Geometry check sheet. Reference: the model listing, model coordinates, mm. Face numbers are marked on the shaded views. A direction names the side the tool comes from. Coordinates: 2 decimals unless noted, no trailing zeros. Loops run counter-clockwise (first coordinate to the right, second up) from the corner with the lowest first, then second, coordinate; pieces in that order, holes last. Notation, with made-up numbers: (10.5, 20.25) - (24.5, 20.25) arc R26 ccw to (24.5, 38.25) - close; hole circle Ø9 at (6, -25.5). An arc over 180 degrees is marked (long way). One line per item, written item: value.
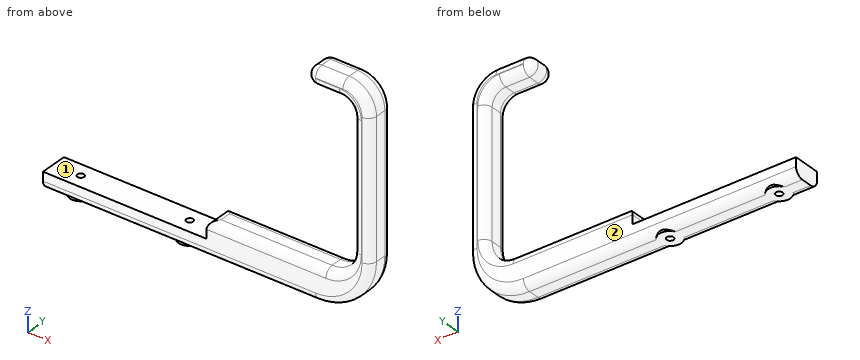
from build123d import *

# Parameters (mm, degrees)
F1_DEPTH = 6.35
F2_R     = 1.575
F3_DEPTH = 7.9385
F4_R     = 3.81
F5_R     = 5.207
F5_R_2   = 1.642683843
F5_R_3   = 1.6124121995
F6_DEPTH = 7.9375


with BuildPart() as f1:
    # F0 (on Front) → F1 (new body, symmetric)
    with BuildSketch(Plane.XZ):
        with BuildLine():
            Line((-18.0305134643, 25.4818645348), (-18.0305134643, 17.5443645348))
            Line((-18.0305134643, 17.5443645348), (108.9694865357, 17.5443645348))
            ThreePointArc((108.9694865357, 17.5443645348), (126.9299987779, 24.9838522926), (134.3694865357, 42.9443645348))
            Line((134.3694865357, 42.9443645348), (134.3694865357, 106.4443645348))
            ThreePointArc((134.3694865357, 106.4443645348), (130.6497426568, 115.4246206558), (121.6694865357, 119.1443645348))
            Line((121.6694865357, 119.1443645348), (108.9694865357, 119.1443645348))
            ThreePointArc((108.9694865357, 119.1443645348), (105.0007365357, 115.1756145348), (108.9694865357, 111.2068645348))
            Line((108.9694865357, 111.2068645348), (120.0819865357, 111.2068645348))
            ThreePointArc((120.0819865357, 111.2068645348), (124.5721145963, 109.3469925953), (126.4319865357, 104.8568645348))
            Line((126.4319865357, 104.8568645348), (126.4319865357, 46.1193645348))
            ThreePointArc((126.4319865357, 46.1193645348), (122.7122426568, 37.1391084137), (113.7319865357, 33.4193645348))
            Line((113.7319865357, 33.4193645348), (58.1694865357, 33.4193645348))
            Line((58.1694865357, 33.4193645348), (58.1694865357, 25.4818645348))
            Line((58.1694865357, 25.4818645348), (-18.0305134643, 25.4818645348))
        make_face()
    extrude(amount=F1_DEPTH, both=True)

    # F2 (on face) → F3 (cut, through all)
    with BuildSketch(Plane.XY.offset(25.4818645348)):
        with Locations((45.4694865357, 0)):
            Circle(F2_R)
        with Locations((-5.3305134643, 0)):
            Circle(F2_R)
    extrude(amount=-F3_DEPTH, mode=Mode.SUBTRACT)

    # F4
    f4_edges = [f1.edges().sort_by_distance(p)[0] for p in [
        (126.431987, 6.35, 75.488115),
        (126.431987, -6.35, 75.488115),
        (124.572115, -6.35, 109.346993),
        (124.572115, 6.35, 109.346993),
        (122.712243, -6.35, 37.139108),
        (122.712243, 6.35, 37.139108),
        (85.950737, 6.35, 33.419365),
        (85.950737, -6.35, 33.419365),
        (58.169487, 0, 33.419365),
        (114.525737, 6.35, 111.206865),
        (114.525737, -6.35, 111.206865),
        (105.000737, -6.35, 115.175615),
        (105.000737, 6.35, 115.175615),
        (115.319487, 6.35, 119.144365),
        (115.319487, -6.35, 119.144365),
        (130.649743, 6.35, 115.424621),
        (134.369487, 6.35, 74.694365),
        (134.369487, -6.35, 74.694365),
        (130.649743, -6.35, 115.424621),
        (126.929999, 6.35, 24.983852),
        (126.929999, -6.35, 24.983852),
        (45.469487, 6.35, 17.544365),
        (45.469487, -6.35, 17.544365),
    ]]
    fillet(f4_edges, radius=F4_R)

    # F5 (on face) → F6 (join, through all)
    with BuildSketch(Plane(origin=(0, 0, 17.5443645348), x_dir=(1, 0, 0), z_dir=(0, 0, -1))):
        with Locations((-5.3305134643, 0)):
            Circle(F5_R)
        with Locations((-5.3305134643, 0)):
            Circle(F5_R_2, mode=Mode.SUBTRACT)
        with Locations((45.4694865357, 0)):
            Circle(F5_R)
        with Locations((45.4694865357, 0)):
            Circle(F5_R_3, mode=Mode.SUBTRACT)
    extrude(amount=-F6_DEPTH)


solid = f1.part
(1) Cross-section at B-B on x = 67.5. Record the cut outline in (y, z).
Reply:
outline: (-6.35, 21.35) arc R3.81 ccw to (-2.54, 17.54) - (2.54, 17.54) arc R3.81 ccw to (6.35, 21.35) - (6.35, 29.61) arc R3.81 ccw to (2.54, 33.42) - (-2.54, 33.42) arc R3.81 ccw to (-6.35, 29.61) - close
(2) Cross-section at C-C on z = 102. Record the cut outline in (x, y).
Reply:
outline: (126.43, -2.54) arc R3.81 ccw to (130.24, -6.35) - (130.56, -6.35) arc R3.81 ccw to (134.37, -2.54) - (134.37, 2.54) arc R3.81 ccw to (130.56, 6.35) - (130.24, 6.35) arc R3.81 ccw to (126.43, 2.54) - close
(3) Material ranges on probe 1 along Z at (x, y) = (41, -2.25); probe 2 along X at (y, z) = (-0.75, 58); probe 3 along Z at (x, y) = (64, -2), recorded low to high. Write a range as from..to.
Reply:
probe 1: 17.54..25.48
probe 2: 126.43..134.37
probe 3: 17.54..33.42
(4) Go/stop test with flat-tipped pins: pin 1 Ø1.5 at (y, z) = (0.5, 78) entering from -X; pin 2 Ø1.5 at (x, y) = (117, -0.5) entering from -Z; pin 3 Ø5 at (x, y) = (3, -1) entering from +Z. Record where each tip stops, or that it passes through.
Reply:
pin 1: x = 126.43
pin 2: z = 18.61
pin 3: z = 25.48
(5) Cross-section at A-A on y = 0. Record the cut outline in (x, z), and give its area (3 significant figures).
Reply:
outline: (-18.03, 17.54) - (-6.91, 17.54) - (-6.91, 25.48) - (-18.03, 25.48) - close; (-3.76, 17.54) - (43.89, 17.54) - (43.89, 25.48) - (-3.76, 25.48) - close; (47.04, 17.54) - (108.97, 17.54) arc R25.4 ccw to (134.37, 42.94) - (134.37, 106.44) arc R12.7 ccw to (121.67, 119.14) - (108.97, 119.14) arc R3.97 ccw to (108.97, 111.21) - (120.08, 111.21) arc R6.35 cw to (126.43, 104.86) - (126.43, 46.12) arc R12.7 cw to (113.73, 33.42) - (61.98, 33.42) arc R3.81 ccw to (58.17, 29.61) - (58.17, 25.48) - (47.04, 25.48) - close
area: 2,480 mm2
(6) Access from +Z, -Z, +X, -X, +Y, -Y to the whole of each face (thin tool, end or side, straight path). Record for the marked faces 1 and 2.
Reply:
face 1: +Z, -X, +Y, -Y
face 2: +Z, -Z, +X, -X, +Y
